Drawing for the job (mm, zero at the part's lowest x, y, z). A direction names the side the tool comes from. Round coordinates to 2 decimals unless told otherwise and drop trailing zeros. Write each loop counter-clockwise with the first axis right and the second up, starting at its lowest first coordinate (ties: lowest second). Pieces come first, ordered by that corner, then holes.
Item 1: Band-saw the part on D-D, the plane x = 30. Write the cut outline in (y, z).
Item 2: Band-saw the part on C-C, the plane y = 5.5. Write the cut outline in (x, z), then the cut area to 3 significant figures.
Item 3: Drop flat-ended pins along their axis: pin 1 Ø5 at (y, z) = (12.5, 17) entering from -X; pin 2 Ø12 at (x, y) = (21, 27) entering from +Z; pin 3 Ø4.5 at (y, z) = (8.5, 63.5) entering from +X; pin 4 Ø1 at (y, z) = (29.5, 30) entering from -X. Give the stop position or say it passes through.
Item 4: Band-saw the part on B-B, the plane x = 19.5. Write the cut outline in (y, z).
Item 5: 3-axis set-ups, long thin cutter, end or side, ignore diameter. For the marked faces 1, 2 and 3: which of +Z, -Z, +X, -X, +Y, -Y reach the whole face in a straight line?
Item 6: Wall check: probe 1 along X at (y, z) = (30, 19.5); probe 2 along Y at (x, z) = (36.5, 32.5); probe 3 along Z at (x, y) = (15, 25). Give the ranges that are in metal, low to high.
Item 7: Band-saw the part on A-A, the plane z = 27. Write the cut outline in (x, y), then the cut area to 3 significant figures.
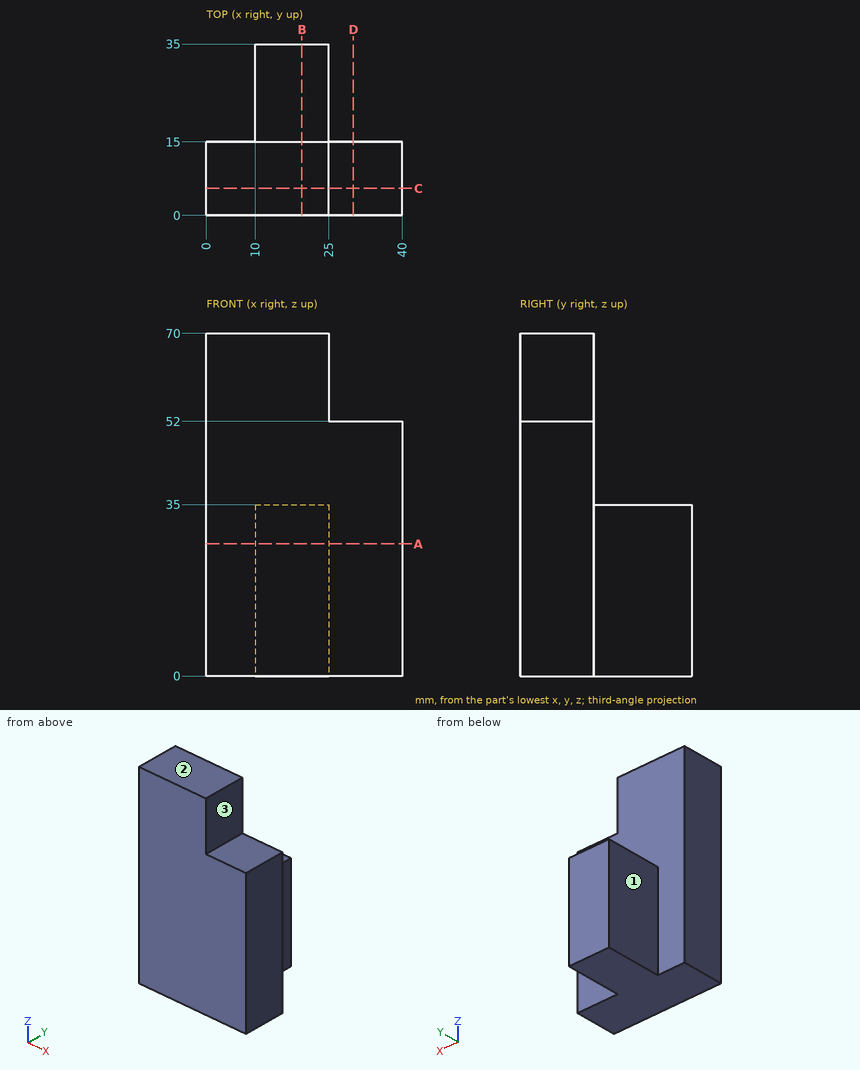
Results:
1. outline: (0, 0) - (15, 0) - (15, 52) - (0, 52) - close
2. outline: (0, 0) - (40, 0) - (40, 52) - (25, 52) - (25, 70) - (0, 70) - close
2. area: 2,530 mm2
3. pin 1: stops at x = 0
3. pin 2: stops at z = 35
3. pin 3: stops at x = 25
3. pin 4: stops at x = 10
4. outline: (0, 0) - (35, 0) - (35, 35) - (15, 35) - (15, 70) - (0, 70) - close
5. face 1: +Z, -Z, -X, +Y
5. face 2: +Z, +X, -X, +Y, -Y
5. face 3: +Z, +X, +Y, -Y
6. probe 1: x = 10 to 25
6. probe 2: y = 0 to 15
6. probe 3: z = 0 to 35
7. outline: (0, 0) - (40, 0) - (40, 15) - (25, 15) - (25, 35) - (10, 35) - (10, 15) - (0, 15) - close
7. area: 900 mm2
